The listing builds one solid part. Answer for the finished solid, in the listing's coordinates (mm). A direction names the side the tool comes from. Coordinates: 2 decimals unless noted, no trailing zeros. Order: outer loops, then holes, each group sorted by start corner. A loop starts at its lowest first (then second) coordinate and runs counter-clockwise, first axis right, second up. Notation, with made-up numbers: (30, 16.25) - (72, 16.25) arc R35 cw to (72, 52.25) - close; hole circle Ø3 at (65, 15.25). An arc over 180 degrees is marked (long way). Use a Markdown table: item, result. Add a question column.
Item 1: A flat-ended cylindrical pin translates along its axis: P1, Ø3.5, axis at x = 83.9, y = 15.18, coming from the +Z side. Find the tip coordinate at first contact, or state that the pin passes through.
Item 2: The part is cut by section B-B, the plane x = -127. Give the vertices of the cut face in (y, z), then the cut area to 3 significant figures.
Item 3: The mould has two halves that part along Y. Classify faces 1 (the flat face through (202.623, 122, 7)), 2 (the flat face through (5, -71.815, 10)), 3 (the flat face through (0, -74.815, 7)): released by +Y, released by -Y, zero draft, split by the parting line, or undercut.
Item 4: The part is cut by section A-A, the plane z = 8.5. Give the vertices of the cut face in (x, y).
Item 5: For faces 4 (the flat face through (199.623, 122, 10)), 5 (the flat face through (-197.377, 128, 7)), determine the directions among +Z, -Z, +X, -X, +Y, -Y from which every point of the face is accessible in a straight line to the end or side of a thin tool.
Item 6: Find the intervals of material crossed by line 1 along X through (y, z) = (283, 8.5); line 2 along Y through (x, z) = (2.5, 11); line 3 along Z through (x, y) = (87.5, -49), in increasing order.
Item 7: The part is cut by section C-C, the plane y = -28.5. Give the vertices of the cut face in (x, z), then the cut area to 3 significant figures.
from build123d import *

# Parameters (mm, degrees)
F0_W      = 400
F0_H      = 400
F1_DEPTH  = 5
F2_R      = 1.5
F2_R_2    = 1.75
F3_DEPTH  = 5.001
F4_R      = 1.5
F5_DEPTH  = 5.001
F6_R      = 1.5
F7_DEPTH  = 5.001
F9_W      = 3
F9_H      = 394
F10_DEPTH = 10
F11_W     = 30
F11_H     = 15
F12_DEPTH = 3
F13_W     = 30
F13_H     = 15
F14_DEPTH = 3


with BuildPart() as f1:
    # F0 (on Top) → F1 (new body)
    with BuildSketch(Plane.XY):
        with Locations((2.6232805103, 125.1846492136)):
            Rectangle(F0_W, F0_H)
    extrude(amount=F1_DEPTH)

    # F2 (on face) → F3 (cut, through all)
    with BuildSketch(Plane.XY.offset(5)):
        with Locations((-158.3767194897, 145.1846492136)):
            Circle(F2_R)
        with Locations((-64.3767194897, 145.1846492136)):
            Circle(F2_R)
        with Locations((-44.3767194897, 145.1846492136)):
            Circle(F2_R)
        with Locations((49.6232805103, 145.1846492136)):
            Circle(F2_R)
        with Locations((69.6232805103, 145.1846492136)):
            Circle(F2_R)
        with Locations((163.6232805103, 145.1846492136)):
            Circle(F2_R)
        with Locations((-44.3767194897, 204.1846492136)):
            Circle(F2_R)
        with Locations((-158.3767194897, 204.1846492136)):
            Circle(F2_R)
        with Locations((49.6232805103, 204.1846492136)):
            Circle(F2_R)
        with Locations((69.6232805103, 204.1846492136)):
            Circle(F2_R)
        with Locations((163.6232805103, 204.1846492136)):
            Circle(F2_R)
        with Locations((-64.3767194897, 204.1846492136)):
            Circle(F2_R)
        with Locations((-173.3767194897, 158.1846492136)):
            Circle(F2_R_2)
        with Locations((-173.3767194897, 191.1846492136)):
            Circle(F2_R_2)
        with Locations((178.6232805103, 158.1846492136)):
            Circle(F2_R_2)
        with Locations((178.6232805103, 191.1846492136)):
            Circle(F2_R_2)
    extrude(amount=-F3_DEPTH, mode=Mode.SUBTRACT)

    # F4 (on face) → F5 (cut, through all)
    with BuildSketch(Plane.XY.offset(5)):
        with Locations((-23.3767194897, 15.1846492136)):
            Circle(F4_R)
        with Locations((-23.3767194897, 59.6346492136)):
            Circle(F4_R)
        with Locations((28.6232805103, 15.1846492136)):
            Circle(F4_R)
        with Locations((28.6232805103, 59.6346492136)):
            Circle(F4_R)
    extrude(amount=-F5_DEPTH, mode=Mode.SUBTRACT)

    # F6 (on face) → F7 (cut, through all)
    with BuildSketch(Plane.XY.offset(5)):
        with Locations((-78.6517194897, 15.1846492136)):
            Circle(F6_R)
        with Locations((-78.6517194897, 59.6346492136)):
            Circle(F6_R)
        with Locations((83.8982805103, 15.1846492136)):
            Circle(F6_R)
        with Locations((83.8982805103, 59.6346492136)):
            Circle(F6_R)
    extrude(amount=-F7_DEPTH, mode=Mode.SUBTRACT)

    # F9 (on face) → F10 (join)
    with BuildSketch(Plane.XY.offset(5)):
        Polygon((-197.3767194897, -71.8153507864), (-197.3767194897, -74.8153507864), (202.6232805103, -74.8153507864), (202.6232805103, -71.8153507864), (199.6232805103, -71.8153507864), (-194.3767194897, -71.8153507864), align=None)
        Polygon((-197.3767194897, 325.1846492136), (-197.3767194897, -71.8153507864), (-194.3767194897, -71.8153507864), (-194.3767194897, 322.1846492136), (-194.3767194897, 325.1846492136), align=None)
        with Locations((201.1232805103, 125.1846492136)):
            Rectangle(F9_W, F9_H)
        Polygon((199.6232805103, 322.1846492136), (202.6232805103, 322.1846492136), (202.6232805103, 325.1846492136), (-194.3767194897, 325.1846492136), (-194.3767194897, 322.1846492136), align=None)
    extrude(amount=F10_DEPTH)

    # F11 (on face) → F12 (cut, through all)
    with BuildSketch(Plane.XZ.offset(74.8153507864)):
        with Locations((0, 22.5)):
            Rectangle(F11_W, F11_H)
    extrude(amount=-F12_DEPTH, mode=Mode.SUBTRACT)

    # F13 (on face) → F14 (cut, through all)
    with BuildSketch(Plane(origin=(0, 325.1846492136, 0), x_dir=(-1, 0, 0), z_dir=(0, 1, 0))):
        with Locations((0, 22.5)):
            Rectangle(F13_W, F13_H)
    extrude(amount=-F14_DEPTH, mode=Mode.SUBTRACT)


solid = f1.part
Solution:
| question | item | result |
|---|---|---|
| 1 | P1 | stops at z = 5 |
| 2 | outline | (-74.82, 0) - (325.18, 0) - (325.18, 15) - (322.18, 15) - (322.18, 5) - (-71.82, 5) - (-71.82, 15) - (-74.82, 15) - close |
| 2 | area | 2,060 mm2 |
| 3 | face 1 | zero draft |
| 3 | face 2 | undercut |
| 3 | face 3 | released by -Y |
| 4 | outline | (-197.38, -74.82) - (202.62, -74.82) - (202.62, 325.18) - (-197.38, 325.18) - close; hole (-194.38, -71.82) - (199.62, -71.82) - (199.62, 322.18) - (-194.38, 322.18) - close |
| 5 | face 4 | +Z |
| 5 | face 5 | +Z, -Z, -X, +Y, -Y |
| 6 | line 1 | x = -197.38 to -194.38, 199.62 to 202.62 |
| 6 | line 2 | y = -74.82 to -71.82, 322.18 to 325.18 |
| 6 | line 3 | z = 0 to 5 |
| 7 | outline | (-197.38, 0) - (202.62, 0) - (202.62, 15) - (199.62, 15) - (199.62, 5) - (-194.38, 5) - (-194.38, 15) - (-197.38, 15) - close |
| 7 | area | 2,060 mm2 |
